Source: CAD feature listing. Evaluate the final solid. Frame: model axes, mm. Give positions to 0.01 mm unless a question says otherwise; leave off trailing zeros. Write each loop counter-clockwise with the first axis right and the second up, starting at its lowest first coordinate (ties: lowest second). Pieces come first, ordered by that corner, then holes. Notation, with made-up numbers: M 23,-17 L 64,-17 A24 cw 64,4 Z; hole C 8,32.25 d7. An arc over 180 degrees is marked long. Use CSV: the item, a comma, the result in double quotes. Start each with the question number.
from build123d import *

# Parameters (mm, degrees)
SKETCH1_W           = 138
SKETCH1_H           = 15
BOSS_EXTRUDE1_DEPTH = 3
SKETCH2_W           = 142
SKETCH2_H           = 19
SKETCH2_W_2         = 138
SKETCH2_H_2         = 15
BOSS_EXTRUDE2_DEPTH = 5


with BuildPart() as part:
    # Sketch1 → Boss-Extrude1 (new body)
    with BuildSketch(Plane(origin=(0, 0, 0), x_dir=(1, 0, 0), z_dir=(0, 1, 0))):
        with Locations((69, 7.5)):
            Rectangle(SKETCH1_W, SKETCH1_H)
    extrude(amount=BOSS_EXTRUDE1_DEPTH)

    # Sketch2 → Boss-Extrude2 (add)
    with BuildSketch(Plane.XZ):
        with Locations((69, -7.5)):
            Rectangle(SKETCH2_W, SKETCH2_H)
        with Locations((69, -7.5)):
            Rectangle(SKETCH2_W_2, SKETCH2_H_2, mode=Mode.SUBTRACT)
    extrude(amount=-BOSS_EXTRUDE2_DEPTH)


solid = part.part
Item 1: Pull-direction query (Z, two-part tool) for faces 1 (the flat face through (68, 2, 2)), 2 (the flat face through (68, 3, -8)), 3 (the flat face through (-2, 2, -8)); classes: released by +Z, released by -Z, zero draft, split by the parting line, or undercut.
Item 2: Section B-B (x = 40). Return the cut outline in (y, z).
Item 3: Material intervals for probe 1 along Z at (x, y) = (63, 3.35); probe 2 along X at (y, z) = (4.85, -9); probe 3 along Y at (x, z) = (130.5, -8.5), sorted ascending.
Item 4: Section A-A (y = 3.9). Return the cut outline in (x, z).
Item 5: Section C-C (z = -7). Return the cut outline in (x, y).
Item 6: Contact query for flat-ended pins moving along their axis: pin 1 Ø3 at (x, z) = (124, -10.5) entering from +Y; pin 2 Ø6 at (x, z) = (52, -6) entering from -Y. Output: stop coordinate, or through.
Output values:
1,face 1,"released by +Z"
1,face 2,"undercut"
1,face 3,"zero draft"
2,outline,"M 0,-17 L 5,-17 L 5,-15 L 3,-15 L 3,0 L 5,0 L 5,2 L 0,2 Z"
3,probe 1,"z = -17 to -15, 0 to 2"
3,probe 2,"x = -2 to 0, 138 to 140"
3,probe 3,"y = 0 to 3"
4,outline,"M -2,-17 L 140,-17 L 140,2 L -2,2 Z; hole M 0,-15 L 138,-15 L 138,0 L 0,0 Z"
5,outline,"M -2,0 L 140,0 L 140,5 L 138,5 L 138,3 L 0,3 L 0,5 L -2,5 Z"
6,pin 1,"stops at y = 3"
6,pin 2,"stops at y = 0"
